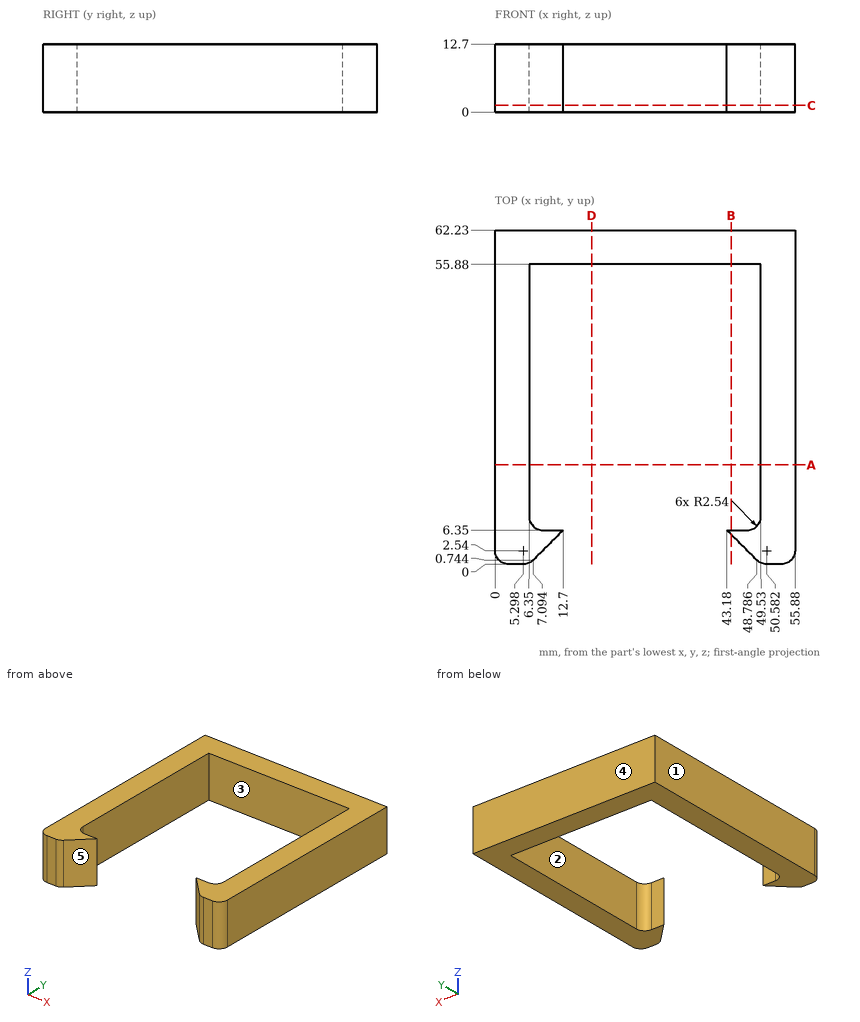
Check sheet for the drawn part. Datum: minimum x, y, z corner. Units: mm. A direction names the side the tool comes from. Round coordinates to 2 decimals unless told otherwise and drop trailing zeros. Loops run counter-clockwise (first coordinate to the right, second up) from the corner with the lowest first, then second, coordinate; pieces in that order, holes last. Notation, with made-up numbers: (87, 40.5) - (113, 40.5) arc R19 cw to (113, 70.5) - close; hole circle Ø10 at (28.25, 51). An arc over 180 degrees is marked (long way). Write each question's results on one line, items separated by ' | '. Start each with the question number.
Q1. Cross-section at B-B on x = 44. Enter the section's corners in (y, z).
Q2. Release check for a two-part mould opening along Y. For the marked faces 3, 4 and 5 record: +Y half, -Y half, draft (parallel to the pull), parting line (faces both ways), or undercut.
Q3. Cross-section at C-C on z = 1.25. Enter the section's corners in (x, y), and give its area (3 significant figures).
Q4. Cross-section at D-D on x = 18. Enter the section's corners in (y, z).
Q5. Cross-section at A-A on y = 18.5. Enter the section's corners in (x, z), and give its area (3 significant figures).
Q6. Access from +Z, -Z, +X, -X, +Y, -Y to the whole of each face (thin tool, end or side, straight path). Record for the marked faces 1 and 2.
Q7. Gauge pin test, flat ends, axial feed: P1, Ø1.5, axis at x = 17.5, z = 5.5, coming from the -Y side; P2, Ø5, axis at x = 10.5, z = 1.5, coming from the -Y side. Record the tip position at first contact, or that the pin passes through.
Q8. Thickness scan on line 1 (X direction, y = 54.5, z = 6.5); line 2 (Y direction, x = 25.5, z = 2); line 3 (Y direction, x = 12, z = 12). Record the ranges inside material, lowest first. Write a range as [from, to].
Answers below:
1) outline: (5.53, 0) - (6.35, 0) - (6.35, 12.7) - (5.53, 12.7) - close; (55.88, 0) - (62.23, 0) - (62.23, 12.7) - (55.88, 12.7) - close
2) face 3: undercut | face 4: +Y half | face 5: -Y half
3) outline: (0, 2.54) arc R2.54 ccw to (2.54, 0) - (5.3, 0) arc R2.54 ccw to (7.09, 0.74) - (12.7, 6.35) - (8.89, 6.35) arc R2.54 cw to (6.35, 8.89) - (6.35, 55.88) - (49.53, 55.88) - (49.53, 8.89) arc R2.54 cw to (46.99, 6.35) - (43.18, 6.35) - (48.79, 0.74) arc R2.54 ccw to (50.58, 0) - (53.34, 0) arc R2.54 ccw to (55.88, 2.54) - (55.88, 62.23) - (0, 62.23) - close | area: 1,100 mm²
4) outline: (55.88, 0) - (62.23, 0) - (62.23, 12.7) - (55.88, 12.7) - close
5) outline: (0, 0) - (6.35, 0) - (6.35, 12.7) - (0, 12.7) - close; (49.53, 0) - (55.88, 0) - (55.88, 12.7) - (49.53, 12.7) - close | area: 161 mm²
6) face 1: +Z, -Z, -X, +Y, -Y | face 2: +Z, -Z
7) P1: stops at y = 55.88 | P2: stops at y = 1.65
8) line 1: x = [0, 6.35], [49.53, 55.88] | line 2: y = [55.88, 62.23] | line 3: y = [5.65, 6.35], [55.88, 62.23]
